Input: part model. Units: mm. Frame: model coordinates. Face numbers are marked on the shaded views. A direction names the side the tool comes from. Give positions to 0.01 mm unless a question says otherwise; leave off trailing zeros. Loops run counter-clockwise (first coordinate to the right, second up) from the corner with the lowest first, then second, coordinate; pieces in that order, holes last. Notation, with made-up numbers: (65, 52.5) - (73, 52.5) arc R11 ccw to (73, 68.5) - close; hole circle Ø3 at (-7.5, 58.25). An arc over 180 degrees is marked (long way). One line per question, with ' | ' between items. Start each with the question number.
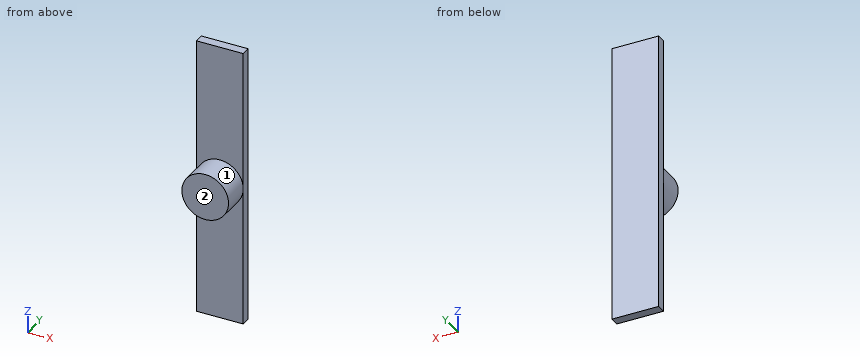
from build123d import *

# Parameters (mm, degrees)
ESQUISSE1_R        = 2.5
BOSS_EXTRU_1_DEPTH = 3
ESQUISSE2_W        = 5
ESQUISSE2_H        = 30
BOSS_EXTRU_2_DEPTH = 1


with BuildPart() as part:
    # Esquisse1 → Boss.-Extru.1 (new body)
    with BuildSketch(Plane(origin=(0, 0, 0), x_dir=(1, 0, 0), z_dir=(0, 1, 0))):
        with Locations(Location((0, 0, 0), (0, 0, 270))):
            Circle(ESQUISSE1_R)
    extrude(amount=BOSS_EXTRU_1_DEPTH)

    # Esquisse2 → Boss.-Extru.2 (add)
    with BuildSketch(Plane(origin=(0, 3, 0), x_dir=(1, 0, 0), z_dir=(0, 1, 0))):
        Rectangle(ESQUISSE2_W, ESQUISSE2_H)
    extrude(amount=BOSS_EXTRU_2_DEPTH)


solid = part.part
Q1. Section A-A, the plane x = 0. Output: boundary loops of the cut face in (y, z).
Q2. Section B-B, the plane y = 0.55. Output: boundary loops of the cut face in (x, z).
Q3. Access query for the marked faces 1 and 2. Directions: +Z, -Z, +X, -X, +Y, -Y. A direction counts if a zero-diameter tool reaches every point of the face in a straight line with its end or side. Return the directions, or none.
Q4. Section C-C, the plane z = -0.5. Output: boundary loops of the cut face in (x, y).
Q5. Section D-D, the plane z = 9. Output: boundary loops of the cut face in (x, y).
Q6. First-contact query: pin 1 (2 mm diameter, centred on x = -0.5, z = 3.5, fed in from -Y). Flat tip, straight axial feed; report the tip coordinate or a pass-through.
Q7. Line query: L1, parallel to Y at x = -2.1, z = -4.25; L2, parallel to Z at x = 0.1, y = 0.3; L3, parallel to X at y = 2.15, z = 2.25. Output: solid intervals per line, ascending. Write a range as from..to.
Solved:
1) outline: (0, -2.5) - (3, -2.5) - (3, -15) - (4, -15) - (4, 15) - (3, 15) - (3, 2.5) - (0, 2.5) - close
2) outline: circle Ø5 at (0, 0)
3) face 1: -Y | face 2: +Z, -Z, +X, -X, -Y
4) outline: (-2.5, 3) - (-2.45, 3) - (-2.45, 0) - (2.45, 0) - (2.45, 3) - (2.5, 3) - (2.5, 4) - (-2.5, 4) - close
5) outline: (-2.5, 3) - (2.5, 3) - (2.5, 4) - (-2.5, 4) - close
6) pin 1: stops at y = 3
7) L1: y = 3..4 | L2: z = -2.5..2.5 | L3: x = -1.09..1.09
